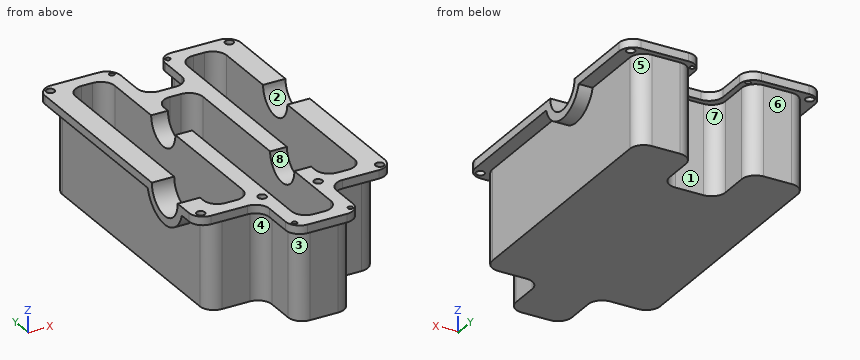
```python
from build123d import *

# Parameters (mm, degrees)
SKETCH1_W           = 70
SKETCH1_H           = 119
BOSS_EXTRUDE1_DEPTH = 35
SKETCH2_R           = 8
CUT_EXTRUDE1_DEPTH  = 8
CUT_EXTRUDE2_DEPTH  = 32
SKETCH4_R           = 7.5
CUT_EXTRUDE3_DEPTH  = 8
SKETCH5_W           = 16
SKETCH5_H           = 20
SKETCH5_W_2         = 23
CUT_EXTRUDE4_DEPTH  = 36
CUT_EXTRUDE5_DEPTH  = 5
SKETCH7_W           = 18
SKETCH7_H           = 32
CUT_EXTRUDE6_DEPTH  = 2
SKETCH8_W           = 32
SKETCH8_H           = 22
CUT_EXTRUDE7_DEPTH  = 2
SKETCH9_W           = 22
SKETCH9_H           = 32
CUT_EXTRUDE8_DEPTH  = 2
SKETCH10_W          = 32
SKETCH10_H          = 18
CUT_EXTRUDE9_DEPTH  = 2
SKETCH11_W          = 25
SKETCH11_H          = 32
CUT_EXTRUDE10_DEPTH = 2
CUT_EXTRUDE11_DEPTH = 5
SKETCH14_W          = 22
SKETCH14_H          = 32
CUT_EXTRUDE12_DEPTH = 2
SKETCH16_W          = 32
SKETCH16_H          = 18
CUT_EXTRUDE13_DEPTH = 2
SKETCH17_W          = 18
SKETCH17_H          = 32
CUT_EXTRUDE14_DEPTH = 2
SKETCH18_W          = 32
SKETCH18_H          = 22
CUT_EXTRUDE15_DEPTH = 2
SKETCH19_W          = 20
SKETCH19_H          = 32
CUT_EXTRUDE16_DEPTH = 2
FILLET1_R           = 5
FILLET3_R           = 5
FILLET4_R           = 5
SKETCH20_R          = 1.5
CUT_EXTRUDE17_DEPTH = 10
SKETCH21_R          = 0.9
CUT_EXTRUDE18_DEPTH = 10
BOSS_EXTRUDE2_DEPTH = 6
BOSS_EXTRUDE3_DEPTH = 6


with BuildPart() as part:
    # Sketch1 → Boss-Extrude1 (new body)
    with BuildSketch(Plane.XY):
        Rectangle(SKETCH1_W, SKETCH1_H)
    extrude(amount=BOSS_EXTRUDE1_DEPTH)

    # Sketch2 → Cut-Extrude1 (cut)
    with BuildSketch(Plane.ZY.offset(35)):
        with Locations((35, -19.5)):
            Circle(SKETCH2_R)
    extrude(amount=-CUT_EXTRUDE1_DEPTH, mode=Mode.SUBTRACT)

    # Sketch3 → Cut-Extrude2 (cut)
    with BuildSketch(Plane.XY.offset(35)):
        Polygon((-27, 54.5), (-13, 54.5), (-13, 27), (-7, 27), (-7, 34.5), (7, 34.5), (7, -12), (13, -12), (13, 54.5), (27, 54.5), (27, -34.5), (13, -34.5), (13, -27), (7, -27), (7, -54.5), (-7, -54.5), (-7, 12), (-13, 12), (-13, -34.5), (-27, -34.5), align=None)
    extrude(amount=-CUT_EXTRUDE2_DEPTH, mode=Mode.SUBTRACT)

    # Sketch4 → Cut-Extrude3 (cut)
    with BuildSketch(Plane(origin=(35, 0, 0), x_dir=(0, 0, -1), z_dir=(1, 0, 0))):
        with Locations((-35, 19.5)):
            Circle(SKETCH4_R)
    extrude(amount=-CUT_EXTRUDE3_DEPTH, mode=Mode.SUBTRACT)

    # Sketch5 → Cut-Extrude4 (cut, through all)
    with BuildSketch(Plane.XY.offset(35)):
        with Locations((0, 49.5)):
            Rectangle(SKETCH5_W, SKETCH5_H)
        with Locations((-23.5, -49.5)):
            Rectangle(SKETCH5_W_2, SKETCH5_H)
        with Locations((23.5, -49.5)):
            Rectangle(SKETCH5_W_2, SKETCH5_H)
    extrude(amount=-CUT_EXTRUDE4_DEPTH, mode=Mode.SUBTRACT)

    # Sketch6 → Cut-Extrude5 (cut)
    with BuildSketch(Plane.ZY.offset(35)):
        with BuildLine():
            Line((32, 59.5), (0, 59.5))
            Line((0, 59.5), (0, -39.5))
            Line((0, -39.5), (32, -39.5))
            Line((32, -39.5), (32, -30.083005244))
            ThreePointArc((32, -30.083005244), (24, -19.5), (32, -8.916994756))
            Line((32, -8.916994756), (32, 59.5))
        make_face()
    extrude(amount=-CUT_EXTRUDE5_DEPTH, mode=Mode.SUBTRACT)

    # Sketch7 → Cut-Extrude6 (cut)
    with BuildSketch(Plane.XZ.offset(39.5)):
        with Locations((-21, 16)):
            Rectangle(SKETCH7_W, SKETCH7_H)
    extrude(amount=-CUT_EXTRUDE6_DEPTH, mode=Mode.SUBTRACT)

    # Sketch8 → Cut-Extrude7 (cut)
    with BuildSketch(Plane.ZY.offset(12)):
        with Locations((16, -48.5)):
            Rectangle(SKETCH8_W, SKETCH8_H)
    extrude(amount=-CUT_EXTRUDE7_DEPTH, mode=Mode.SUBTRACT)

    # Sketch9 → Cut-Extrude8 (cut)
    with BuildSketch(Plane.XZ.offset(59.5)):
        with Locations((1, 16)):
            Rectangle(SKETCH9_W, SKETCH9_H)
    extrude(amount=-CUT_EXTRUDE8_DEPTH, mode=Mode.SUBTRACT)

    # Sketch10 → Cut-Extrude9 (cut)
    with BuildSketch(Plane(origin=(12, 0, 0), x_dir=(0, 0, -1), z_dir=(1, 0, 0))):
        with Locations((-16, -48.5)):
            Rectangle(SKETCH10_W, SKETCH10_H)
    extrude(amount=-CUT_EXTRUDE9_DEPTH, mode=Mode.SUBTRACT)

    # Sketch11 → Cut-Extrude10 (cut)
    with BuildSketch(Plane.XZ.offset(39.5)):
        with Locations((22.5, 16)):
            Rectangle(SKETCH11_W, SKETCH11_H)
    extrude(amount=-CUT_EXTRUDE10_DEPTH, mode=Mode.SUBTRACT)

    # Sketch13 → Cut-Extrude11 (cut)
    with BuildSketch(Plane(origin=(35, 0, 0), x_dir=(0, 0, -1), z_dir=(1, 0, 0))):
        with BuildLine():
            Line((-32, 59.5), (0, 59.5))
            Line((0, 59.5), (0, -37.5))
            Line((0, -37.5), (-32, -37.5))
            Line((-32, -37.5), (-32, 9.437694101))
            ThreePointArc((-32, 9.437694101), (-24.5, 19.5), (-32, 29.562305899))
            Line((-32, 29.562305899), (-32, 59.5))
        make_face()
    extrude(amount=-CUT_EXTRUDE11_DEPTH, mode=Mode.SUBTRACT)

    # Sketch14 → Cut-Extrude12 (cut)
    with BuildSketch(Plane(origin=(0, 59.5, 0), x_dir=(1, 0, 0), z_dir=(0, 1, 0))):
        with Locations((19, -16)):
            Rectangle(SKETCH14_W, SKETCH14_H)
    extrude(amount=-CUT_EXTRUDE12_DEPTH, mode=Mode.SUBTRACT)

    # Sketch16 → Cut-Extrude13 (cut)
    with BuildSketch(Plane.ZY.offset(-8)):
        with Locations((16, 48.5)):
            Rectangle(SKETCH16_W, SKETCH16_H)
    extrude(amount=-CUT_EXTRUDE13_DEPTH, mode=Mode.SUBTRACT)

    # Sketch17 → Cut-Extrude14 (cut)
    with BuildSketch(Plane(origin=(0, 39.5, 0), x_dir=(1, 0, 0), z_dir=(0, 1, 0))):
        with Locations((1, -16)):
            Rectangle(SKETCH17_W, SKETCH17_H)
    extrude(amount=-CUT_EXTRUDE14_DEPTH, mode=Mode.SUBTRACT)

    # Sketch18 → Cut-Extrude15 (cut)
    with BuildSketch(Plane(origin=(-8, 0, 0), x_dir=(0, 0, -1), z_dir=(1, 0, 0))):
        with Locations((-16, 48.5)):
            Rectangle(SKETCH18_W, SKETCH18_H)
    extrude(amount=-CUT_EXTRUDE15_DEPTH, mode=Mode.SUBTRACT)

    # Sketch19 → Cut-Extrude16 (cut)
    with BuildSketch(Plane(origin=(0, 59.5, 0), x_dir=(1, 0, 0), z_dir=(0, 1, 0))):
        with Locations((-20, -16)):
            Rectangle(SKETCH19_W, SKETCH19_H)
    extrude(amount=-CUT_EXTRUDE16_DEPTH, mode=Mode.SUBTRACT)

    # Fillet1
    fillet1_edges = [part.edges().sort_by_distance(p)[0] for p in [
        (-27, -34.5, 19),
        (-27, 54.5, 19),
        (-13, 54.5, 19),
        (-7, 34.5, 19),
        (7, 34.5, 19),
        (13, 54.5, 19),
        (27, 54.5, 19),
        (27, -34.5, 19),
        (13, -34.5, 19),
        (7, -54.5, 19),
        (-7, -54.5, 19),
        (-13, -34.5, 19),
    ]]
    fillet(fillet1_edges, radius=FILLET1_R)

    # Fillet3
    fillet3_edges = [part.edges().sort_by_distance(p)[0] for p in [
        (-30, -37.5, 16),
        (-10, -37.5, 16),
        (-10, -57.5, 16),
        (10, -57.5, 16),
        (10, -37.5, 16),
        (30, -37.5, 16),
        (30, 57.5, 16),
        (10, 57.5, 16),
        (10, 37.5, 16),
        (-10, 37.5, 16),
        (-10, 57.5, 16),
        (-30, 57.5, 16),
    ]]
    fillet(fillet3_edges, radius=FILLET3_R)

    # Fillet4
    fillet4_edges = [part.edges().sort_by_distance(p)[0] for p in [
        (-35, -39.5, 33.5),
        (-12, -39.5, 33.5),
        (-12, -59.5, 33.5),
        (12, -59.5, 33.5),
        (12, -39.5, 33.5),
        (35, -39.5, 33.5),
        (8, 59.5, 33.5),
        (8, 39.5, 33.5),
        (-8, 39.5, 33.5),
        (-8, 59.5, 33.5),
        (-35, 59.5, 33.5),
        (35, 59.5, 33.5),
    ]]
    fillet(fillet4_edges, radius=FILLET4_R)

    # Sketch20 → Cut-Extrude17 (cut)
    with BuildSketch(Plane.XY.offset(35)):
        with Locations((-32, 56.5)):
            Circle(SKETCH20_R)
        with Locations((32, 56.5)):
            Circle(SKETCH20_R)
        with Locations((32, -36.5)):
            Circle(SKETCH20_R)
        with Locations((-32, -36.5)):
            Circle(SKETCH20_R)
        with Locations((-10, -36.5)):
            Circle(SKETCH20_R)
        with Locations((10, -36.5)):
            Circle(SKETCH20_R)
    extrude(amount=-CUT_EXTRUDE17_DEPTH, mode=Mode.SUBTRACT)

    # Sketch21 → Cut-Extrude18 (cut)
    with BuildSketch(Plane.XY.offset(35)):
        with Locations((-10, 56.5)):
            Circle(SKETCH21_R)
        with Locations((10, 56.5)):
            Circle(SKETCH21_R)
        with Locations((10, -56.5)):
            Circle(SKETCH21_R)
        with Locations((-10, -56.5)):
            Circle(SKETCH21_R)
    extrude(amount=-CUT_EXTRUDE18_DEPTH, mode=Mode.SUBTRACT)

    # Sketch22 → Boss-Extrude2 (add)
    with BuildSketch(Plane.ZY.offset(13)):
        with BuildLine():
            Line((35, 27), (3, 27))
            Line((3, 27), (3, 12))
            Line((3, 12), (35, 12))
            ThreePointArc((35, 12), (27.5, 19.5), (35, 27))
        make_face()
    extrude(amount=-BOSS_EXTRUDE2_DEPTH)

    # Sketch24 → Boss-Extrude3 (add)
    with BuildSketch(Plane.ZY.offset(-7)):
        with BuildLine():
            Line((35, -12), (3, -12))
            Line((3, -12), (3, -27))
            Line((3, -27), (35, -27))
            ThreePointArc((35, -27), (27.5, -19.5), (35, -12))
        make_face()
    extrude(amount=-BOSS_EXTRUDE3_DEPTH)


solid = part.part
```
Source: CAD feature listing. Evaluate the final solid. Frame: model axes, mm. Face numbers are marked on the shaded views. A direction names the side the tool comes from. Round coordinates to 2 decimals unless told otherwise and drop trailing zeros. Loops run counter-clockwise (first coordinate to the right, second up) from the corner with the lowest first, then second, coordinate; pieces in that order, holes last. Notation, with made-up numbers: M -28.75,16 L -18.75,16 A11 ccw -18.75,36 Z; hole C 41.25,86 d11. An arc over 180 degrees is marked long. Use a Markdown table: item, result. Add a question column.
1. Reachability of the marked faces 4, 5, 6, 7 and 8 from +Z, -Z, +X, -X, +Y, -Y: full face, straight path, thin tool, end or side. Return the list, or none.
2. Contact query for flat-ended pins moving along their axis: P1, Ø8, axis at x = 20, z = 19, coming from the +Y side; P2, Ø7, axis at x = -1, y = -6, coming from the +Z side; P3, Ø9.5, axis at y = -5.5, z = 19, coming from the +X side. Output: stop coordinate, or through.
3. Section query C-C on z = 20. Give the number of separate pieces and of enclosed holes in the cut face, then the cut area to 3 significant figures.
4. Section query B-B on y = -47. Return the cut outline in (x, z).
5. Section query A-A on x = 32. Return the cut outline in (y, z), then the cut area to 3 significant figures.
6. Section query D-D on x = -32. Return the cut outline in (y, z).
7. Line query: line 1 (X direction, y = 48, z = 17.5); line 2 (X direction, y = -25, z = 25); line 3 (Y direction, x = 1, z = 27). Output: solid intervals per line, ascending.
8. Mould query, pull axis X, two halves, no side actions, for the marked faces 1, 2 and 3. Classes: pulls with the +X half, pulls with the -X half, needs draft (parallel to the pull), parting line crosses it, or undercut.
Reported:
| question | item | result |
|---|---|---|
| 1 | face 4 | -Z, -X, -Y |
| 1 | face 5 | -Z, +X, +Y |
| 1 | face 6 | -Z, +X, -X, +Y |
| 1 | face 7 | -Z, +Y |
| 1 | face 8 | +Z |
| 2 | P1 | stops at y = 57.5 |
| 2 | P2 | stops at z = 3 |
| 2 | P3 | stops at x = 30 |
| 3 | separate pieces | 1 |
| 3 | enclosed holes | 3 |
| 3 | area | 2,000 mm² |
| 4 | outline | M -12,32 L -10,32 L -10,0 L 10,0 L 10,32 L 12,32 L 12,35 L 7,35 L 7,3 L -7,3 L -7,35 L -12,35 Z |
| 5 | outline | M -39.08,32 L -38,32 L -38,35 L -39.08,35 Z; M -35,32 L 9.44,32 A10.5 ccw 29.56,32 L 55,32 L 55,35 L 27,35 A7.5 cw 12,35 L -35,35 Z; M 58,32 L 59.08,32 L 59.08,35 L 58,35 Z |
| 5 | area | 299 mm² |
| 6 | outline | M -39.08,32 L -38,32 L -38,35 L -39.08,35 Z; M -35,32 L -30.08,32 A11 ccw -8.92,32 L 55,32 L 55,35 L -11.5,35 A8 cw -27.5,35 L -35,35 Z; M 58,32 L 59.08,32 L 59.08,35 L 58,35 Z |
| 7 | line 1 | x = -30 to -27, -13 to -10, 10 to 13, 27 to 30 |
| 7 | line 2 | x = -30 to -27, -13 to -7, 7 to 13, 27 to 30 |
| 7 | line 3 | y = -57.5 to -54.5, 34.5 to 37.5 |
| 8 | face 1 | undercut |
| 8 | face 2 | needs draft |
| 8 | face 3 | pulls with the -X half |
